The figure shows three views and two pictorial views of one solid part (mm, origin at its lowest corner). Answer the questions. Coordinates: 2 decimals unless noted, no trailing zeros. Order: outer loops, then holes, each group sorted by start corner. A loop starts at its lowest first (then second) coordinate and runs counter-clockwise, first axis right, second up. Notation, with made-up numbers: (-17, 63.5) - (17, 63.5) arc R26 cw to (17, 81.5) - close; hole circle Ø6 at (47.5, -29.75). An arc over 180 degrees is marked (long way). Use one line per item in the form item = value. Start each with the question number.
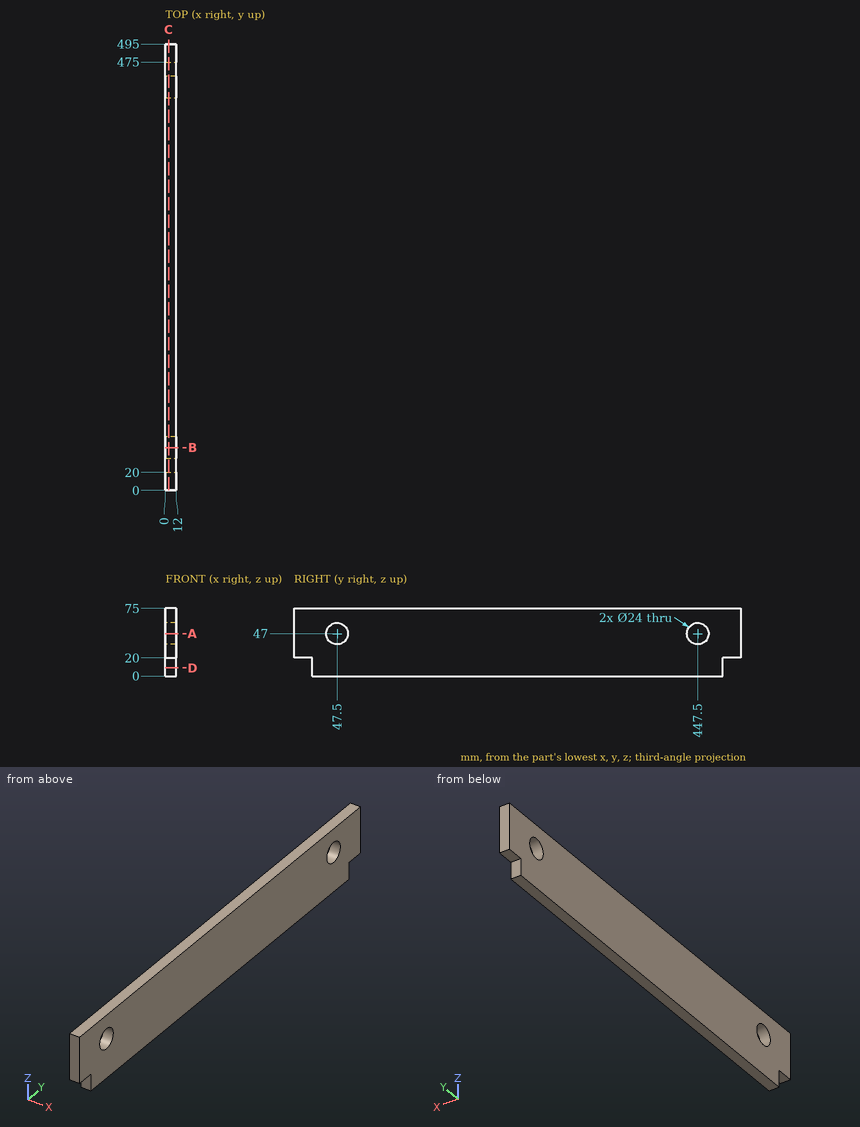
Q1. A cutting plane is placed at A-A (z = 47). Give the vertices of the cut face in (x, y).
Q2. A cutting plane is placed at D-D (z = 9). Give the vertices of the cut face in (x, y), then the cut area to 3 significant figures.
Q3. Given P1, Ø3.5, axis at x = 7, y = 481.5, coming from the -Z side; P2, Ø5, axis at y = 294.5, z = 8, coming from the -X side, each flat-ended and moving along its own axis, determine where each tip first touches the part or whether it passes through.
Q4. A cutting plane is placed at C-C (x = 3.5). Give the vertices of the cut face in (y, z), then the cut area to 3 significant figures.
Q5. A cutting plane is placed at B-B (y = 47.5). Give the vertices of the cut face in (x, z).
Q6. Consider probe 1 along Z at (x, y) = (7.5, 47.5); probe 2 along Y at (x, z) = (1.75, 57); probe 3 along Y at (x, z) = (3.5, 40.5). Determine where each line is inside the solid, lowest interval first.
Result sheet:
q1.outline = (0, 0) - (12, 0) - (12, 35.5) - (0, 35.5) - close; (0, 59.5) - (12, 59.5) - (12, 435.5) - (0, 435.5) - close; (0, 459.5) - (12, 459.5) - (12, 495) - (0, 495) - close
q2.outline = (0, 20) - (12, 20) - (12, 475) - (0, 475) - close
q2.area = 5,460 mm^2
q3.P1 = 20
q3.P2 = 0
q4.outline = (0, 20) - (20, 20) - (20, 0) - (475, 0) - (475, 20) - (495, 20) - (495, 75) - (0, 75) - close; hole circle Ø24 at (47.5, 47); hole circle Ø24 at (447.5, 47)
q4.area = 35,400 mm^2
q5.outline = (0, 0) - (12, 0) - (12, 35) - (0, 35) - close; (0, 59) - (12, 59) - (12, 75) - (0, 75) - close
q6.probe_1 = 0 to 35, 59 to 75
q6.probe_2 = 0 to 40.87, 54.13 to 440.87, 454.13 to 495
q6.probe_3 = 0 to 37.41, 57.59 to 437.41, 457.59 to 495
